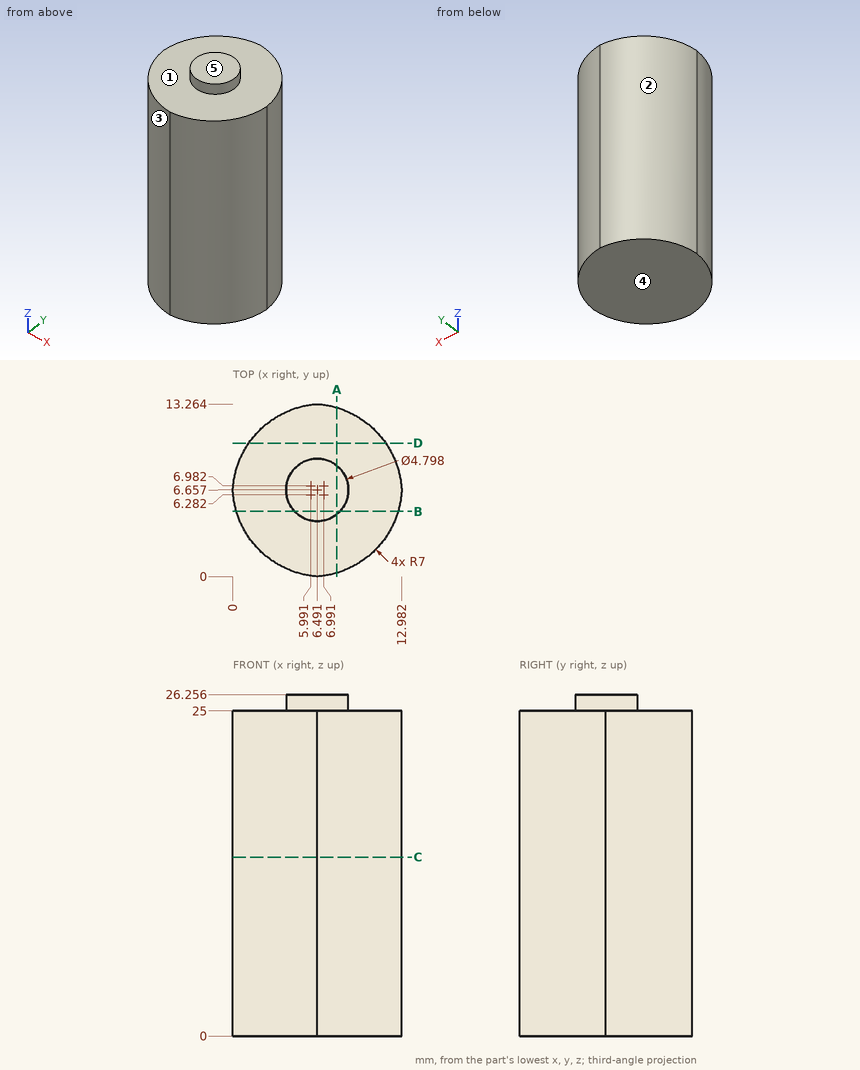
Check sheet for the drawn part. Datum: minimum x, y, z corner. Units: mm. A direction names the side the tool comes from. Round coordinates to 2 decimals unless told otherwise and drop trailing zeros. Write each loop counter-clockwise with the first axis right and the second up, starting at its lowest first coordinate (ties: lowest second). Pieces come first, ordered by that corner, then holes. Notation, with made-up numbers: (57.25, 27) - (69.25, 27) arc R18 ccw to (69.25, 58) - close; hole circle Ø7 at (20, 61). An arc over 180 degrees is marked (long way). Write each question's results on one line, items separated by ' | '.
(1) Sectioned sample at C-C, the plane z = 13.75. Enter the section's corners in (x, y) (1 decimal), plus the area to 3 significant figures.
Computed:
outline: (0, 6.6) arc R7 ccw to (6.5, 0) arc R7 ccw to (13, 6.6) arc R7 ccw to (6.5, 13.3) arc R7 ccw to start | area: 131 mm^2
(2) Set-up check for the marked faces 1 and 2: record each of +Z, -Z, +X, -X, +Y, -Y from which the full face is reachable in a straight line by a thin tool's end or side.
Computed:
face 1: +Z | face 2: +Z, -Z, -X, +Y
(3) Sectioned sample at B-B, the plane y = 5. Enter the section's corners in (x, z) (1 decimal), plus the area to 3 significant figures.
Computed:
outline: (0.3, 0) - (12.7, 0) - (12.7, 25) - (8.2, 25) - (8.2, 26.3) - (4.8, 26.3) - (4.8, 25) - (0.3, 25) - close | area: 315 mm^2
(4) Draft check along Z on the marked faces 3, 4 and 5. Enter one of: pulls with the +Z half, pulls with the -Z half, needs draft (parallel to the pull), parting line crosses it, or undercut.
Computed:
face 3: needs draft | face 4: pulls with the -Z half | face 5: pulls with the +Z half
(5) Sectioned sample at D-D, the plane y = 10.25. Enter the section's corners in (x, z) (1 decimal).
Computed:
outline: (1.2, 0) - (11.8, 0) - (11.8, 25) - (1.2, 25) - close
(6) Thickness scan on probe 1 along Z at (x, y) = (2.5, 7); probe 2 along Y at (x, z) = (4, 6.75) (1 decimal); probe 3 along X at (y, z) = (9.25, 19.5). Record the ranges inside material, lowest first. Write a range as from..to.
Computed:
probe 1: z = 0..25 | probe 2: y = 0.7..12.6 | probe 3: x = 0.65..12.33
(7) Sectioned sample at A-A, the plane x = 8. Enter the section's corners in (y, z).
Computed:
outline: (0.28, 0) - (12.99, 0) - (12.99, 25) - (8.52, 25) - (8.52, 26.26) - (4.79, 26.26) - (4.79, 25) - (0.28, 25) - close
(8) Depth check by flat-ended pin: pin 1 Ø6 at (x, z) = (11.5, 5.5) entering from +Y; pin 2 Ø1 at (x, z) = (4, 4.5) entering from -Y; pin 3 Ø3 at (y, z) = (9.5, 13.5) entering from -X (1 decimal). Enter the tip coordinate at first touch or a pass-through.
Computed:
pin 1: stops at y = 12.82 | pin 2: stops at y = 0.44 | pin 3: stops at x = 0.2
